Autodesk Inventor part; units mm, degrees
ref_plane "YZ Plane" through (0, 0, 0) normal (1, 0, 0) x (0, 1, 0)
ref_plane "XZ Plane" through (0, 0, 0) normal (0, 1, 0) x (-1, 0, 0)
ref_plane "XY Plane" through (0, 0, 0) normal (0, 0, 1) x (1, 0, 0)
sketch "Sketch1" plane through (0, 0, 0) normal (0, 0, 1) x (1, 0, 0)
  line L0 (0, 0) -> (23.2, 0)
  line L1 (23.2, 0) -> (23.2, -60)
  line L2 (23.2, -60) -> (0, -60)
  line L3 (0, -60) -> (0, 0)
  dimension "d0" = 23.2
  dimension "d1" = 60
extrude "Extrusion1" add sketch "Sketch1" along normal blind 8
sketch "Sketch2" plane through (0, 0, 8) normal (0, 0, 1) x (1, 0, 0)
  line L0 (23.2, 0) -> (0, 0)
  line L1 (2.325, -3) -> (20.875, -3)
  line L2 (20.875, -3) -> (20.875, -57)
  line L3 (20.875, -57) -> (2.325, -57)
  line L4 (2.325, -57) -> (2.325, -3)
  line L5 (0, 0) -> (23.2, 0)
  line L6 (23.2, 0) -> (23.2, -60)
  line L7 (23.2, -60) -> (0, -60)
  line L8 (0, -60) -> (0, 0)
  dimension "d8" = 3
  dimension "d9" = 3
  dimension "d10" = 2.325
  dimension "d11" = 2.325
extrude "Extrusion2" cut sketch "Sketch2" against normal blind 5.5 contours L1 L2 L3 L4
sketch "Sketch3" plane through (0, -60, 0) normal (-1, 0, 0) x (0, 0, 1)
  circle A0 centre (2, 57) radius 0.5
  line L0 (0, 60) -> (8, 60)
  line L1 (0, 60) -> (0, 0)
  circle A1 centre (2, 3) radius 0.5
  line L2 (0, 0) -> (8, 0)
  dimension "d16" = 1
  dimension "d17" = 3
  dimension "d21" = 1
  dimension "d22" = 2
  dimension "d23" = 3
  dimension "d24" = 2
extrude "Extrusion3" cut sketch "Sketch3" against normal blind 25
sketch "Sketch4" plane through (0, 0, 8) normal (0, 0, 1) x (1, 0, 0)
  line L0 (2.325, -57) -> (2.325, -3)
  circle A0 centre (1.5, -1.5) radius 1
  line L1 (20.875, -57) -> (2.325, -57)
  line L2 (20.875, -3) -> (20.875, -57)
  line L3 (2.325, -3) -> (20.875, -3)
  line L4 (20.875, -3) -> (20.875, -4.1486)
  circle A1 centre (21.7, -1.5) radius 1
  circle A2 centre (21.7, -58.5) radius 1
  circle A3 centre (1.5, -58.5) radius 1
  line L5 (0, -60) -> (23.2, -60)
  line L6 (23.2, -60) -> (23.2, 0)
  line L7 (23.2, 0) -> (0, 0)
  line L8 (0, 0) -> (0, -60)
  dimension "d27" = 2
  dimension "d29" = 2
  dimension "d31" = 2
  dimension "d32" = 2
  dimension "d34" = 1.5
  dimension "d35" = 1.5
  dimension "d36" = 1.5
  dimension "d37" = 1.5
  dimension "d38" = 1.5
  dimension "d39" = 1.5
  dimension "d40" = 1.5
  dimension "d41" = 1.5
extrude "Extrusion4" add sketch "Sketch4" along normal blind 1.5 contours A0 | A1 | A2 | A3
sketch "Sketch6" plane through (0, 0, 2.5) normal (0, 0, 1) x (1, 0, 0)
  line L0 (2.325, -3) -> (20.875, -3)
  line L1 (20.875, -57) -> (2.325, -57)
  line L2 (2.325, -18.125) -> (20.875, -18.125)
  line L3 (20.875, -51.875) -> (2.325, -51.875)
  line L4 (2.325, -51.875) -> (2.325, -18.125)
  line L5 (23.2, -60) -> (23.2, 0)
  line L6 (20.875, -18.125) -> (20.875, -51.875)
  line L7 (2.325, -57) -> (2.325, -3)
  line L8 (2.325, -3) -> (20.875, -3)
  line L9 (20.875, -3) -> (20.875, -18.125)
  line L10 (20.875, -18.125) -> (2.325, -18.125)
  line L11 (2.325, -18.125) -> (2.325, -3)
  line L12 (2.325, -51.875) -> (20.875, -51.875)
  line L13 (20.875, -51.875) -> (20.875, -57)
  line L14 (20.875, -57) -> (2.325, -57)
  line L15 (2.325, -57) -> (2.325, -51.875)
  point P0 (0, 0)
  dimension "d46" = 15.125
  dimension "d47" = 5.125
  dimension "d49" = 20.875
extrude "Extrusion5" add sketch "Sketch6" along normal blind 5.5 contours L0 L9 L2 L7 | L3 L13 L1 L7
properties part number "BaseBluetooth"
Model file for the job. Use its own axes, mm. A direction names the side the tool comes from. Give positions to 0.01 mm unless a question says otherwise; leave off trailing zeros. Write each loop counter-clockwise with the first axis right and the second up, starting at its lowest first coordinate (ties: lowest second). Pieces come first, ordered by that corner, then holes. Notation, with made-up numbers: (-23.75, 11.5) -> (-6.75, 11.5) arc R26 cw to (-6.75, 31.5) -> close; hole circle Ø2 at (9, -2.75). An arc over 180 degrees is marked (long way). Use CSV: the item, a comma, the result in double quotes. Start each with the question number.
1) Pin check, flat tips, straight feed: P1, Ø12, axis at x = 7, y = -33.5, coming from the +Z side; P2, Ø2, axis at x = 14.5, y = -33, coming from the -Z side; P3, Ø7, axis at x = 17, y = -26, coming from the +Z side. Stop position of each tip, or through.
2) Two-plate mould, pull along X, no slides. Class faces 3 (the flat face through (11, -35, 2.5)), 4 (the cylindrical face through (2.04, -59.34, 8.74)), 5 (the flat face through (23.2, -30, 4)), 6 (the flat face through (12, -60, 4)): released by +X, released by -X, zero draft, split by the parting line, or undercut.
3) Cut at D-D on x = 21.7. List the corners of the cut face in (y, z), plus the area to 3 significant figures.
4) Cut at B-B on z = 4. List the corners of the cut face in (x, y) (3 decimals).
5) Tool access for faces 1 (the cylindrical face through (1.283, -0.524, 8.74)), 2 (the cylindrical face through (11.4, -2.7, 1.6)): list every direction of +Z, -Z, +X, -X, +Y, -Y with a clear straight run to the whole face (end or side of a thin tool).
6) Cut at C-C on y = -58.5. List the corners of the cut face in (x, z).
7) Drill centre lines: L1, parallel to Y at x = 11.25, z = 2; L2, parallel to Z at x = 14.5, y = -57; L3, parallel to Y at x = 11.5, z = 5.5 (3 decimals). Where is each one in solid material? Low to high.
8) Cut at A-A on x = 12.75. List the corners of the cut face in (y, z) (3 decimals), plus the area to 3 significant figures.
Final values:
1,P1,"stops at z = 8"
1,P2,"stops at z = 0"
1,P3,"stops at z = 2.5"
2,face 3,"undercut"
2,face 4,"undercut"
2,face 5,"released by +X"
2,face 6,"zero draft"
3,outline,"(-60, 0) -> (0, 0) -> (0, 8) -> (-0.5, 8) -> (-0.5, 9.5) -> (-2.5, 9.5) -> (-2.5, 8) -> (-57.5, 8) -> (-57.5, 9.5) -> (-59.5, 9.5) -> (-59.5, 8) -> (-60, 8) -> close; hole circle Ø1 at (-57, 2); hole circle Ø1 at (-3, 2)"
3,area,"484 mm2"
4,outline,"(0, -60) -> (23.2, -60) -> (23.2, 0) -> (0, 0) -> close; hole (2.325, -51.875) -> (20.875, -51.875) -> (20.875, -18.125) -> (2.325, -18.125) -> close"
5,face 1,"+Z"
5,face 2,"+X, -X"
6,outline,"(0, 0) -> (23.2, 0) -> (23.2, 8) -> (22.7, 8) -> (22.7, 9.5) -> (20.7, 9.5) -> (20.7, 8) -> (2.5, 8) -> (2.5, 9.5) -> (0.5, 9.5) -> (0.5, 8) -> (0, 8) -> close"
7,L1,"y = -60 to -57.5, -56.5 to -3.5, -2.5 to 0"
7,L2,"z = 0 to 1.5, 2.5 to 8"
7,L3,"y = -60 to -51.875, -18.125 to 0"
8,outline,"(-60, 0) -> (0, 0) -> (0, 8) -> (-18.125, 8) -> (-18.125, 2.5) -> (-51.875, 2.5) -> (-51.875, 8) -> (-60, 8) -> close; hole circle Ø1 at (-57, 2); hole circle Ø1 at (-3, 2)"
8,area,"293 mm2"
